Build history of the part. All positions in model axes, mm. Face numbers are marked on the shaded views. A direction names the side the tool comes from. Round coordinates to 2 decimals unless told otherwise and drop trailing zeros. Order: outer loops, then holes, each group sorted by start corner. A loop starts at its lowest first (then second) coordinate and runs counter-clockwise, first axis right, second up. Notation, with made-up numbers: M -17,-34.75 L 29,-34.75 A4 ccw 29,-30.75 Z; hole C 49.25,73.25 d11. An arc over 180 degrees is marked long. Use CSV: the item, a comma, the result in double quotes.
from build123d import *

# Parameters (mm, degrees)
SKETCH1_R                                = 38.1
OD_DON_T_CARE_DEPTH                      = 63.5
SKETCH2_R                                = 3.175
F_2X_1_4_THROUGH_HOLE_DEPTH              = 50.8
SKETCH3_W                                = 25.4
SKETCH3_H                                = 50.927
SLOT_DEPTH                               = 50.8
SKETCH4_R                                = 7.9375
F_5_8_THROUGH_HOLE_DEPTH                 = 75.140268103
SKETCH5_OUTSIDE_W                        = 103.216
SKETCH5_OUTSIDE_H                        = 103.216
SKETCH5_OUTSIDE_W_2                      = 63.5
SKETCH5_OUTSIDE_H_2                      = 71.842048968
FLAT_SURFACE_FOR_3_4_LONG_SHOULDER_DEPTH = 25.4


with BuildPart() as part:
    # Sketch1 → OD Don't Care (new body)
    with BuildSketch(Plane.XY):
        Circle(SKETCH1_R)
    extrude(amount=OD_DON_T_CARE_DEPTH)

    # Sketch2 → 2x 1/4" Through Hole (cut, symmetric)
    with BuildSketch(Plane(origin=(0, 0, 0), x_dir=(0, 0, -1), z_dir=(1, 0, 0))):
        with Locations(Location((-50.8, 0, 0), (0, 0, 180))):
            Circle(SKETCH2_R)
    extrude(amount=F_2X_1_4_THROUGH_HOLE_DEPTH, both=True, mode=Mode.SUBTRACT)

    # Sketch3 → Slot (cut, symmetric)
    with BuildSketch(Plane(origin=(0, 0, 0), x_dir=(1, 0, 0), z_dir=(0, 1, 0))):
        with Locations((0, -38.0365)):
            Rectangle(SKETCH3_W, SKETCH3_H)
    extrude(amount=SLOT_DEPTH, both=True, mode=Mode.SUBTRACT)

    # Sketch4 → 5/8" Through Hole (cut, through all)
    with BuildSketch(Plane.XY.offset(12.573)):
        Circle(SKETCH4_R)
    extrude(amount=-F_5_8_THROUGH_HOLE_DEPTH, mode=Mode.SUBTRACT)

    # Sketch5 outside → Flat Surface for 3/4" Long Shoulder (cut)
    with BuildSketch(Plane.XY.offset(63.5)):
        Rectangle(SKETCH5_OUTSIDE_W, SKETCH5_OUTSIDE_H)
        Rectangle(SKETCH5_OUTSIDE_W_2, SKETCH5_OUTSIDE_H_2, mode=Mode.SUBTRACT)
    extrude(amount=-FLAT_SURFACE_FOR_3_4_LONG_SHOULDER_DEPTH, mode=Mode.SUBTRACT)


solid = part.part
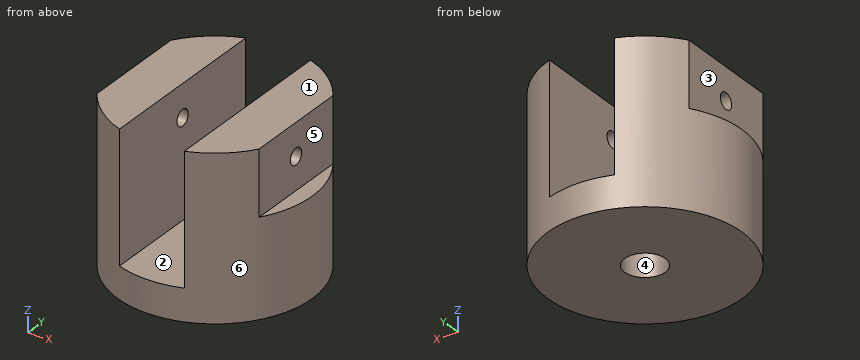
(1) Cut at C-C, the plane y = 0. Count the separate pieces of the cut face and the enclosed holes in it, and give its area (3 significant figures).
Answer block:
separate pieces,"4"
enclosed holes,"0"
area,"2,780 mm²"
(2) Cut at D-D, the plane z = 50.8. Give the cut face in (x, y) (3 decimals), and give its area (3 significant figures).
Answer block:
outline,"M -31.75,-21.061 A38.1 ccw -12.7,-35.921 L -12.7,-3.175 L -31.75,-3.175 Z; M -31.75,3.175 L -12.7,3.175 L -12.7,35.921 A38.1 ccw -31.75,21.061 Z; M 12.7,-35.921 A38.1 ccw 31.75,-21.061 L 31.75,-3.175 L 12.7,-3.175 Z; M 12.7,3.175 L 31.75,3.175 L 31.75,21.061 A38.1 ccw 12.7,35.921 Z"
area,"2,060 mm²"
(3) Tool access for the marked faces 1, 2 and 3: list every direction of +Z, -Z, +X, -X, +Y, -Y with a clear straight run to the whole face (end or side of a thin tool).
Answer block:
face 1,"+Z, +X, -X, +Y, -Y"
face 2,"+Z, +Y, -Y"
face 3,"+Z, -X, +Y, -Y"
(4) Drop flat-ended pins along their axis: pin 1 (6 mm diameter, centred on y = -6, z = 23.5, fed in from -X); pin 2 (8 mm diameter, centred on y = -12, z = 17, fed in from +X); pin 3 (1.5 mm diameter, centred on x = 9.5, y = -10.5, fed in from +Z). Give the stop position or say it passes through.
Answer block:
pin 1,"stops at x = -37.98"
pin 2,"stops at x = 37.25"
pin 3,"stops at z = 12.57"
(5) Two-plate mould, pull along Y, no slides. Class the marked faces 4, 5 and 6: released by +Y, released by -Y, zero draft, split by the parting line, or undercut.
Answer block:
face 4,"undercut"
face 5,"zero draft"
face 6,"split by the parting line"
(6) Cut at A-A, the plane x = 0. Give the cut face in (y, z), and give its area (3 significant figures).
Answer block:
outline,"M -38.1,0 L -7.94,0 L -7.94,12.57 L -38.1,12.57 Z; M 7.94,0 L 38.1,0 L 38.1,12.57 L 7.94,12.57 Z"
area,"758 mm²"
(7) Cut at B-B, the plane z = 40.5. Give the cut face in (x, y).
Answer block:
outline,"M -31.75,-21.06 A38.1 ccw -12.7,-35.92 L -12.7,35.92 A38.1 ccw -31.75,21.06 Z; M 12.7,-35.92 A38.1 ccw 31.75,-21.06 L 31.75,21.06 A38.1 ccw 12.7,35.92 Z"
(8) Wall check: line 1 (X direction, y = -7.5, z = 46); line 2 (Y direction, x = -20.5, z = 50.8) (3 decimals). Give the ranges that are in metal, low to high. Write a range as from..to.
Answer block:
line 1,"x = -31.75..-12.7, 12.7..31.75"
line 2,"y = -32.115..-3.175, 3.175..32.115"
